Design review of the part built by this model. Coordinates are the model's own, in mm. A direction names the side the tool comes from. Coordinates: 2 decimals unless noted, no trailing zeros. Loops run counter-clockwise (first coordinate to the right, second up) from the corner with the lowest first, then second, coordinate; pieces in that order, holes last. Notation, with made-up numbers: (75.25, 47.25) -> (131.25, 47.25) arc R20 cw to (131.25, 56.25) -> close; hole circle Ø11 at (82.25, 17). An arc over 180 degrees is marked (long way). Use CSV: the item, a comma, the result in double quotes.
```python
from build123d import *

# Parameters (mm, degrees)
SKETCH1_R           = 4.50215
SKETCH1_R_2         = 3.1115
BOSS_EXTRUDE2_DEPTH = 15.367
BOSS_EXTRUDE3_DEPTH = 3.0988
BOSS_EXTRUDE4_DEPTH = 6.2484


with BuildPart() as part:
    # Sketch1 → Boss-Extrude2 (new body)
    with BuildSketch(Plane.XY):
        Circle(SKETCH1_R)
        Circle(SKETCH1_R_2, mode=Mode.SUBTRACT)
    extrude(amount=BOSS_EXTRUDE2_DEPTH)

    # Sketch2 → Boss-Extrude3 (add)
    with BuildSketch(Plane.XY.offset(15.367)):
        Polygon((3.759424156, 1.886920364), (1.324060129, 3.992568499), (-1.886920364, 3.759424156), (-3.992568499, 1.324060129), (-3.759424156, -1.886920364), (-1.324060129, -3.992568499), (1.886920364, -3.759424156), (3.992568499, -1.324060129), align=None)
    extrude(amount=BOSS_EXTRUDE3_DEPTH)

    # Sketch3 → Boss-Extrude4 (add)
    with BuildSketch(Plane.XY.offset(18.4658)):
        Polygon((-2.318447564, 3.843004124), (-4.35680427, 1.078024282), (-3.843004124, -2.318447564), (-1.078024282, -4.35680427), (2.318447564, -3.843004124), (4.35680427, -1.078024282), (3.843004124, 2.318447564), (1.078024282, 4.35680427), align=None)
    extrude(amount=BOSS_EXTRUDE4_DEPTH)


solid = part.part
```
Item 1: To check wall thickness, follow line 1 along Y through (x, z) = (0, 8); line 2 along Z through (x, y) = (2.5, -3.25); line 3 along X through (y, z) = (0.5, 12.5). State the ranges of each line that lie inside material, in increasing order.
Checked values:
line 1,"-4.5 to -3.11, 3.11 to 4.5"
line 2,"0 to 15.37, 18.47 to 24.71"
line 3,"-4.47 to -3.07, 3.07 to 4.47"
Item 2: Add section A-A (x = 0). Give the boundary of the cut face in (y, z).
Checked values:
outline,"(-4.5, 0) -> (-3.11, 0) -> (-3.11, 15.37) -> (3.11, 15.37) -> (3.11, 0) -> (4.5, 0) -> (4.5, 15.37) -> (3.9, 15.37) -> (3.9, 18.47) -> (4.19, 18.47) -> (4.19, 24.71) -> (-4.19, 24.71) -> (-4.19, 18.47) -> (-3.9, 18.47) -> (-3.9, 15.37) -> (-4.5, 15.37) -> close"
Item 3: Add section C-C (z = 5). Give the boundary of the cut face in (x, y).
Checked values:
outline,"circle Ø9 at (0, 0); hole circle Ø6.22 at (0, 0)"
Item 4: Add section B-B (y = 2.75). Give the boundary of the cut face in (x, z), then the cut area to 3 significant figures.
Checked values:
outline,"(-3.56, 0) -> (-1.46, 0) -> (-1.46, 15.37) -> (1.46, 15.37) -> (1.46, 0) -> (3.56, 0) -> (3.56, 15.37) -> (2.76, 15.37) -> (2.76, 18.47) -> (3.26, 18.47) -> (3.26, 24.71) -> (-3.12, 24.71) -> (-3.12, 18.47) -> (-2.76, 18.47) -> (-2.76, 15.37) -> (-3.56, 15.37) -> close"
area,"122 mm^2"
Item 5: Machinability: for faces 4 (the face through (-2.48, -3.323, 21.546)), 5 (the face through (2.48, 3.323, 21.546)), 6 (the face through (2.559, 2.925, 16.895)), 7 (the face through (-0.259, 3.878, 16.895)), which of the approach directions +Z, -Z, +X, -X, +Y, -Y give a long, thin tool a straight path to every point of the face, cutting with its end or side? Answer none if there is none.
Checked values:
face 4,"+Z, -X, -Y"
face 5,"+Z, +X, +Y"
face 6,"+X, +Y"
face 7,"-X, +Y"
Item 6: Draft analysis for pull direction Y (two halves, no side actions). For faces 1 (the face through (0, 0, 15.367)), 2 (the face through (0.259, -3.878, 16.895)), 3 (the face through (-0.596, 4.104, 21.546)), state which applies: pulls with the +Y half, pulls with the -Y half, needs draft (parallel to the pull), parting line crosses it, or undercut.
Checked values:
face 1,"undercut"
face 2,"pulls with the -Y half"
face 3,"pulls with the +Y half"
Item 7: Clearance check with flat-ended pins moving along their axes: pin 1 (2 mm diameter, centred on y = -1.5, z = 8, fed in from -X); pin 2 (1.9 mm diameter, centred on x = -1, y = 1.5, fed in from -Z). State where each tip first meets the part, or that it passes through.
Checked values:
pin 1,"x = -4.47"
pin 2,"z = 15.37"
